```python
from build123d import *

# Parameters (mm, degrees)
SKETCH_1_R      = 6.48
EXTRUDE_1_DEPTH = 3.9
FILLET_1_R      = 1


with BuildPart() as part:
    # Эскиз1 → Бобышка-Вытянуть1 (new body)
    with BuildSketch(Plane(origin=(0, 0, 0), x_dir=(1, 0, 0), z_dir=(0, 1, 0))):
        Polygon((0.679491924, 10), (8.320508076, 5.588457268), (9, 4.411542732), (9, -4.411542732), (8.320508076, -5.588457268), (0.679491924, -10), (-0.679491924, -10), (-8.320508076, -5.588457268), (-9, -4.411542732), (-9, 4.411542732), (-8.320508076, 5.588457268), (-0.679491924, 10), align=None)
        with Locations(Location((0, 0, 0), (0, 0, 270))):
            Circle(SKETCH_1_R, mode=Mode.SUBTRACT)
    extrude(amount=EXTRUDE_1_DEPTH)

    # Скругление1
    fillet_1_edges = [part.edges().sort_by_distance(p)[0] for p in [
        (-8.660254038, 0, -5),
        (0, 0, -10),
        (8.660254038, 0, -5),
        (8.660254038, 0, 5),
        (0, 0, 10),
        (-8.660254038, 0, 5),
    ]]
    fillet(fillet_1_edges, radius=FILLET_1_R)


solid = part.part
```
Source: CAD feature listing. Evaluate the final solid. Frame: model axes, mm. Coordinates: 2 decimals unless noted, no trailing zeros. Write each loop counter-clockwise with the first axis right and the second up, starting at its lowest first coordinate (ties: lowest second). Pieces come first, ordered by that corner, then holes. Notation, with made-up numbers: M 70.25,-20 L 112.25,-20 A29 cw 112.25,18 Z; hole C -29.5,-25 d1. An arc over 180 degrees is marked long. Answer as a JSON object with one key per item and string values.
1. Cut plane C-C on z = 0. Output: boundary loops of the cut face in (x, y), plus the area to 3 significant figures.
Evaluation:
{"outline": "M -9,0 L -6.48,0 L -6.48,3.9 L -9,3.9 Z; M 6.48,0 L 9,0 L 9,3.9 L 6.48,3.9 Z", "area": "19.7 mm^2"}
2. Ray query, L1, parallel to X at y = 1.65, z = 0; L2, parallel to Z at x = 0.25, y = 2.65; L3, parallel to Z at x = 5.25, y = 1.5. Return the intervals inside material, ascending.
Evaluation:
{"L1": "-9 to -6.48, 6.48 to 9", "L2": "-10 to -6.48, 6.48 to 10", "L3": "-7.36 to -3.8, 3.8 to 7.36"}
3. Cut plane B-B on y = 1.9. Output: boundary loops of the cut face in (x, z).
Evaluation:
{"outline": "M -9,-4.41 L -8.32,-5.59 L -0.68,-10 L 0.68,-10 L 8.32,-5.59 L 9,-4.41 L 9,4.41 L 8.32,5.59 L 0.68,10 L -0.68,10 L -8.32,5.59 L -9,4.41 Z; hole C 0,0 d12.96"}
4. Cut plane A-A on x = 0. Output: boundary loops of the cut face in (y, z), plus the area to 3 significant figures.
Evaluation:
{"outline": "M 0,-9 A1 ccw 1,-10 L 3.9,-10 L 3.9,-6.48 L 0,-6.48 Z; M 0,6.48 L 3.9,6.48 L 3.9,10 L 1,10 A1 ccw 0,9 Z", "area": "27.0 mm^2"}
5. Draft query along X for faces 1 (the flat face through (9, 2, 0)), 2 (the flat face through (0, 2, 10)), 3 (the flat face through (-8.665, 2.43, -4.992)), 4 (the cylindrical face through (-6.326, 1.923, -1.405)). Return one class per face: released by +X, released by -X, zero draft, split by the parting line, or undercut.
Evaluation:
{"face 1": "released by +X", "face 2": "zero draft", "face 3": "released by -X", "face 4": "undercut"}
6. Cut plane D-D on x = -3.5. Output: boundary loops of the cut face in (y, z), plus the area to 3 significant figures.
Evaluation:
{"outline": "M 0,-8.37 L 3.9,-8.37 L 3.9,-5.45 L 0,-5.45 Z; M 0,5.45 L 3.9,5.45 L 3.9,8.37 L 0,8.37 Z", "area": "22.8 mm^2"}
